Read the model definition and answer for the solid it produces. Units are mm, in the model's axes. A direction names the side the tool comes from. Round coordinates to 2 decimals unless told otherwise and drop trailing zeros. Write each loop counter-clockwise with the first axis right and the second up, starting at its lowest first coordinate (ties: lowest second). Pieces come first, ordered by that corner, then holes. Notation, with made-up numbers: (75, 50) -> (107, 50) arc R27 ccw to (107, 87) -> close; hole circle Ø11 at (64, 7.5). An arc over 180 degrees is marked (long way). Return JSON: item names as keys, results as strings. Group by question number.
(1) For faces 4 (the flat face through (49, 27, -44)), 5 (the flat face through (39, 16, -14.9)), 6 (the flat face through (93, 14, -42)), 7 (the flat face through (8, 6.4, -32)), 8 (the flat face through (72, 6.4, -7)), determine the directions among +Z, -Z, +X, -X, +Y, -Y from which every point of the face is accessible in a straight line to the end or side of a thin tool.
(2) The mould has two halves that part along Y. Classify faces 1 (the flat face through (0, 5, -33)), 2 (the flat face through (8, 14, -21.5)), 3 (the flat face through (50, 25, -7)): released by +Y, released by -Y, zero draft, split by the parting line, or undercut.
(3) A cutting plane is placed at A-A on z = -77. Give the vertices of the cut face in (x, y), then the cut area to 3 significant figures.
(4) A cutting plane is placed at D-D on y = 14. State how many separate pieces and enclosed holes the cut face has, then the cut area to 3 significant figures.
(5) Straight lines are drawn through the part: line 1 (X direction, y = 22, z = -9); line 2 (Z direction, x = 75, y = 5.5); line 3 (Y direction, x = 95.5, z = -25). For each, find the intervals that lie inside material, in ascending order.
(6) A cutting plane is placed at C-C on y = 32. Give the vertices of the cut face in (x, z), then the cut area to 4 significant figures.
(7) Given pin 1 (16.5 mm diameter, centred on x = 29, z = -6, fed in from -Y); pin 2 (5 mm diameter, centred on x = 77, z = -45, fed in from +Y); pin 3 (1.5 mm diameter, centred on x = 49.5, z = -70.5, fed in from -Y); pin 4 (2.5 mm diameter, centred on x = 48, z = -20, fed in from +Y), each flat-ended and moving along its own axis, determine where each tip first touches the part or whether it passes through.
(8) A cutting plane is placed at B-B on x = 30. Give the vertices of the cut face in (y, z).
```python
from build123d import *

# Parameters (mm, degrees)
CROQUIS1_W              = 100
CROQUIS1_H              = 49
SALIENTE_EXTRUIR1_DEPTH = 40
CROQUIS2_W              = 70
CROQUIS2_H              = 29
CORTAR_EXTRUIR1_DEPTH   = 35
CORTAR_EXTRUIR2_DEPTH   = 14.9
CORTAR_EXTRUIR4_DEPTH   = 119.325821358
CROQUIS6_W              = 20.5
CROQUIS6_H              = 16.2
CORTAR_EXTRUIR6_DEPTH   = 119.325821358
CROQUIS7_W              = 58
CROQUIS7_H              = 18
SALIENTE_EXTRUIR2_DEPTH = 16
CROQUIS8_W              = 54
CROQUIS8_H              = 14
CORTAR_EXTRUIR7_DEPTH   = 16
ENVOLVER2_START         = -2.5
ENVOLVER2_DEPTH         = 2.5
CROQUIS11_W             = 75
CROQUIS11_H             = 10
SALIENTE_EXTRUIR3_DEPTH = 51
CROQUIS12_W             = 67
CROQUIS12_H             = 52
CORTAR_EXTRUIR8_DEPTH   = 5
CROQUIS13_W             = 71
CROQUIS13_H             = 1.5
CORTAR_EXTRUIR9_DEPTH   = 54
CROQUIS14_W             = 20
CROQUIS14_H             = 12
CORTAR_EXTRUIR10_DEPTH  = 5
CORTAR_EXTRUIR11_REACH  = 148.969
CROQUIS5_W              = 20.5
CROQUIS5_H              = 16.2


# Read off the part's stored shape, not the designer's step: Envolver2
with BuildPart() as part:
    # Croquis1 → Saliente-Extruir1 (new body)
    with BuildSketch(Plane(origin=(0, 0, 0), x_dir=(1, 0, 0), z_dir=(0, 1, 0))):
        with Locations((50, 24.5)):
            Rectangle(CROQUIS1_W, CROQUIS1_H)
    extrude(amount=SALIENTE_EXTRUIR1_DEPTH)

    # Croquis2 → Cortar-Extruir1 (cut)
    with BuildSketch(Plane(origin=(0, 40, 0), x_dir=(1, 0, 0), z_dir=(0, 1, 0))):
        with Locations((50, 29.5)):
            Rectangle(CROQUIS2_W, CROQUIS2_H)
    extrude(amount=-CORTAR_EXTRUIR1_DEPTH, mode=Mode.SUBTRACT)

    # Croquis3 → Cortar-Extruir2 (cut)
    with BuildSketch(Plane.XY):
        Polygon((15, 5), (15, 25), (85, 25), (85, 5), (100, 5), (100, 40), (0, 40), (0, 5), align=None)
    extrude(amount=-CORTAR_EXTRUIR2_DEPTH, mode=Mode.SUBTRACT)

    # Croquis4 → Cortar-Extruir4 (cut, through all)
    with BuildSketch(Plane.ZY):
        Polygon((-44, 25), (-19, 25), (-19, 5), (-14.9, 5), (-14.9, 40), (-44, 40), align=None)
    extrude(amount=-CORTAR_EXTRUIR4_DEPTH, mode=Mode.SUBTRACT)

    # Croquis6 → Cortar-Extruir6 (cut, through all)
    with BuildSketch(Plane(origin=(100, 0, 0), x_dir=(0, 0, -1), z_dir=(1, 0, 0))):
        with Locations((31.75, 14.5)):
            Rectangle(CROQUIS6_W, CROQUIS6_H)
    extrude(amount=-CORTAR_EXTRUIR6_DEPTH, mode=Mode.SUBTRACT)

    # Croquis7 → Saliente-Extruir2 (add)
    with BuildSketch(Plane(origin=(0, 5, 0), x_dir=(1, 0, 0), z_dir=(0, 1, 0))):
        with Locations((50, 35)):
            Rectangle(CROQUIS7_W, CROQUIS7_H)
    extrude(amount=SALIENTE_EXTRUIR2_DEPTH)

    # Croquis8 → Cortar-Extruir7 (cut)
    with BuildSketch(Plane(origin=(0, 21, 0), x_dir=(1, 0, 0), z_dir=(0, 1, 0))):
        with Locations((50, 35)):
            Rectangle(CROQUIS8_W, CROQUIS8_H)
    extrude(amount=-CORTAR_EXTRUIR7_DEPTH, mode=Mode.SUBTRACT)

    # Envolver2 outline → Envolver2 (cut)
    # profile 1 of 3: a face of its own
    with BuildSketch(Plane(origin=(0, 5, 0), x_dir=(1, 0, 0), z_dir=(0, 1, 0)).offset(ENVOLVER2_START)):
        with BuildLine():
            add(Edge.make_bspline(
                [(44.845927513, 22.682039813), (44.880502524, 22.681581101), (44.94779002, 22.680688388), (45.045978034, 22.678103561), (45.138406194, 22.671034857), (45.225422346, 22.663758255), (45.306894242, 22.652117669), (45.382891805, 22.638865253), (45.453428219, 22.622573117), (45.519399834, 22.604194379), (45.582065701, 22.58175166), (45.642294727, 22.553081251), (45.700763218, 22.518735345), (45.757273689, 22.477750733), (45.813128977, 22.432374893), (45.865885411, 22.37921084), (45.918377238, 22.321807714), (45.967578278, 22.25830401), (46.01447324, 22.191680732), (46.054376208, 22.120908747), (46.088223994, 22.047966819), (46.117214563, 21.973058038), (46.136979973, 21.894799291), (46.154181469, 21.814812457), (46.162464556, 21.732060085), (46.163897144, 21.676148523), (46.164618555, 21.647993057)],
                knots=[0, 0, 0, 0, 0.054369818, 0.105810783, 0.1543913, 0.200099433, 0.243069893, 0.283740822, 0.321360744, 0.356845277, 0.391373506, 0.42587086, 0.461574928, 0.497826917, 0.535543491, 0.574581255, 0.615459073, 0.657779879, 0.700797841, 0.743450957, 0.785305491, 0.827181235, 0.869502041, 0.912065543, 0.955718718, 1, 1, 1, 1], degree=3))
            Line((44.845927513, 22.682039813), (43.424314244, 22.682039813))
            Line((43.424314244, 22.682039813), (42.805172718, 18.976839617))
            Line((42.805172718, 18.976839617), (43.469342719, 18.976839617))
            Line((43.469342719, 18.976839617), (43.718607489, 20.469211918))
            Line((43.718607489, 20.469211918), (44.603095383, 20.469211918))
            Line((44.603095383, 20.469211918), (45.04292709, 18.976839617))
            Line((45.04292709, 18.976839617), (45.752929645, 18.976839617))
            Line((45.752929645, 18.976839617), (45.28977962, 20.548011749))
            add(Edge.make_bspline(
                [(46.164618555, 21.647993057), (46.164091676, 21.617670303), (46.163039403, 21.5571103), (46.151744736, 21.467468845), (46.13622668, 21.379126232), (46.112503265, 21.292592771), (46.082048693, 21.207680933), (46.044780457, 21.124441143), (46.001130757, 21.043108672), (45.951712013, 20.9635574), (45.895224481, 20.887990565), (45.830214645, 20.819272615), (45.758276279, 20.757071565), (45.678885267, 20.701205138), (45.592072867, 20.652370985), (45.497799172, 20.610367641), (45.396617343, 20.574987864), (45.325850603, 20.557119534), (45.28977962, 20.548011749)],
                knots=[0, 0, 0, 0, 0.059520551, 0.118873267, 0.177208837, 0.235565778, 0.294841411, 0.354222133, 0.414510544, 0.476000381, 0.538010758, 0.599455515, 0.661405537, 0.724496825, 0.78978963, 0.856706752, 0.926961053, 1, 1, 1, 1], degree=3))
        make_face()
        with BuildLine():
            add(Edge.make_bspline(
                [(44.743809366, 21.03528417), (44.778129381, 21.03600119), (44.843652036, 21.0373701), (44.937526666, 21.044910102), (45.022020151, 21.059216882), (45.097465695, 21.079213334), (45.164300411, 21.104537257), (45.221481868, 21.136836672), (45.270624581, 21.17399479), (45.32077283, 21.232312946), (45.36864261, 21.310567266), (45.413007527, 21.407196099), (45.438530205, 21.507321555), (45.442292151, 21.574957755), (45.444162962, 21.608593141)],
                knots=[0, 0, 0, 0, 0.099664188, 0.190275618, 0.273183536, 0.348129931, 0.416633313, 0.480054439, 0.538277477, 0.594505454, 0.702244126, 0.80362549, 0.902343236, 1, 1, 1, 1], degree=3))
            Line((44.743809366, 21.03528417), (43.812684837, 21.03528417))
            Line((43.812684837, 21.03528417), (43.993602816, 22.115967561))
            Line((43.993602816, 22.115967561), (44.735768567, 22.115967561))
            add(Edge.make_bspline(
                [(45.444162962, 21.608593141), (45.443321191, 21.636863214), (45.441681994, 21.691914124), (45.421908744, 21.770970842), (45.392768442, 21.844328967), (45.35019923, 21.909220717), (45.300609579, 21.965653441), (45.246923641, 22.013950522), (45.187891151, 22.050903022), (45.122329195, 22.077622199), (45.046506806, 22.09459194), (44.957252302, 22.107151834), (44.85196106, 22.115045121), (44.776255138, 22.115646142), (44.735768567, 22.115967561)],
                knots=[0, 0, 0, 0, 0.084973229, 0.165470167, 0.24404472, 0.32176826, 0.397881214, 0.469968558, 0.538528016, 0.606605512, 0.682202732, 0.771959831, 0.878046995, 1, 1, 1, 1], degree=3))
        make_face(mode=Mode.SUBTRACT)
    # profile 2 of 3: a face of its own
    with BuildSketch(Plane(origin=(0, 5, 0), x_dir=(1, 0, 0), z_dir=(0, 1, 0)).offset(ENVOLVER2_START)):
        Polygon((46.976739258, 22.682039813), (46.357597732, 18.976839617), (48.79395984, 18.976839617), (48.892057588, 19.542911869), (47.113432841, 19.542911869), (47.285505941, 20.572134146), (48.696666171, 20.572134146), (48.78913536, 21.138206398), (47.379583289, 21.138206398), (47.54281151, 22.115967561), (49.257109864, 22.115967561), (49.355207612, 22.682039813), align=None)
    # profile 3 of 3: a face of its own
    with BuildSketch(Plane(origin=(0, 5, 0), x_dir=(1, 0, 0), z_dir=(0, 1, 0)).offset(ENVOLVER2_START)):
        Polygon((50.984273497, 22.682039813), (49.96148386, 22.682039813), (49.342342334, 18.976839617), (49.858561632, 18.976839617), (50.417397165, 22.321007936), (50.952914381, 18.976839617), (51.313946257, 18.976839617), (52.891551028, 22.350758892), (52.327086936, 18.976839617), (52.991256936, 18.976839617), (53.611202541, 22.682039813), (52.559466028, 22.682039813), (51.387921608, 20.172506434), align=None)
    extrude(amount=ENVOLVER2_DEPTH, mode=Mode.SUBTRACT)

    # Croquis11 → Saliente-Extruir3 (add)
    with BuildSketch(Plane(origin=(0, 0, -49), x_dir=(-1, 0, 0), z_dir=(0, 0, -1))):
        with Locations((-50, 35)):
            Rectangle(CROQUIS11_W, CROQUIS11_H)
    extrude(amount=SALIENTE_EXTRUIR3_DEPTH)

    # Croquis12 → Cortar-Extruir8 (cut)
    with BuildSketch(Plane(origin=(0, 40, 0), x_dir=(1, 0, 0), z_dir=(0, 1, 0))):
        with Locations((50, 70)):
            Rectangle(CROQUIS12_W, CROQUIS12_H)
    extrude(amount=-CORTAR_EXTRUIR8_DEPTH, mode=Mode.SUBTRACT)

    # Croquis13 → Cortar-Extruir9 (cut)
    with BuildSketch(Plane.XY.offset(-44)):
        with Locations((50, 37.5)):
            Rectangle(CROQUIS13_W, CROQUIS13_H)
    extrude(amount=-CORTAR_EXTRUIR9_DEPTH, mode=Mode.SUBTRACT)

    # Croquis14 → Cortar-Extruir10 (cut)
    with BuildSketch(Plane(origin=(0, 35, 0), x_dir=(1, 0, 0), z_dir=(0, 1, 0))):
        with Locations((50.5, 81)):
            Rectangle(CROQUIS14_W, CROQUIS14_H)
    extrude(amount=-CORTAR_EXTRUIR10_DEPTH, mode=Mode.SUBTRACT)

    # Croquis5 → Cortar-Extruir11 (cut, up to next)
    with BuildSketch(Plane.XY, mode=Mode.PRIVATE) as cortar_extruir11_sk1:
        with Locations((27.5, 14.5)):
            Rectangle(CROQUIS5_W, CROQUIS5_H)
    cortar_extruir11_tool1 = extrude(cortar_extruir11_sk1.sketch, amount=-CORTAR_EXTRUIR11_REACH, mode=Mode.PRIVATE) & part.part
    # Croquis5 → Cortar-Extruir11 (cut, up to next)
    with BuildSketch(Plane.XY, mode=Mode.PRIVATE) as cortar_extruir11_sk2:
        with Locations((50, 14.5)):
            Rectangle(CROQUIS5_W, CROQUIS5_H)
    cortar_extruir11_tool2 = extrude(cortar_extruir11_sk2.sketch, amount=-CORTAR_EXTRUIR11_REACH, mode=Mode.PRIVATE) & part.part
    # Croquis5 → Cortar-Extruir11 (cut, up to next)
    with BuildSketch(Plane.XY, mode=Mode.PRIVATE) as cortar_extruir11_sk3:
        with Locations((72.5, 14.5)):
            Rectangle(CROQUIS5_W, CROQUIS5_H)
    cortar_extruir11_tool3 = extrude(cortar_extruir11_sk3.sketch, amount=-CORTAR_EXTRUIR11_REACH, mode=Mode.PRIVATE) & part.part
    add(cortar_extruir11_tool1.solids().sort_by_distance((27.5, 14.5, 0))[0], mode=Mode.SUBTRACT)
    add(cortar_extruir11_tool2.solids().sort_by_distance((50, 14.5, 0))[0], mode=Mode.SUBTRACT)
    add(cortar_extruir11_tool3.solids().sort_by_distance((72.5, 14.5, 0))[0], mode=Mode.SUBTRACT)


solid = part.part
```
Checks:
{
 "1": {"face 4": "+Y", "face 5": "+X, -X, +Y", "face 6": "+X", "face 7": "-X", "face 8": "+Z"},
 "2": {"face 1": "zero draft", "face 2": "undercut", "face 3": "released by +Y"},
 "3": {"outline": "(12.5, 30) -> (40.5, 30) -> (40.5, 35) -> (16.5, 35) -> (16.5, 36.75) -> (14.5, 36.75) -> (14.5, 38.25) -> (16.5, 38.25) -> (16.5, 40) -> (12.5, 40) -> close; (60.5, 30) -> (87.5, 30) -> (87.5, 40) -> (83.5, 40) -> (83.5, 38.25) -> (85.5, 38.25) -> (85.5, 36.75) -> (83.5, 36.75) -> (83.5, 35) -> (60.5, 35) -> close", "area": "309 mm^2"},
 "4": {"separate pieces": "7", "enclosed holes": "1", "area": "1,050 mm^2"},
 "5": {"line 1": "x = 15 to 17.25, 37.75 to 39.75, 60.25 to 62.25, 82.75 to 85", "line 2": "z = -49 to -42, -28 to -26, -14.9 to 0", "line 3": "y = 0 to 6.4, 22.6 to 25"},
 "6": {"outline": "(0, -49) -> (12.5, -49) -> (12.5, -100) -> (87.5, -100) -> (87.5, -49) -> (100, -49) -> (100, -44) -> (0, -44) -> close; hole (40.5, -87) -> (60.5, -87) -> (60.5, -75) -> (40.5, -75) -> close", "area": "4,085 mm^2"},
 "7": {"pin 1": "stops at y = 0", "pin 2": "stops at y = 35", "pin 3": "stops at y = 30", "pin 4": "stops at y = 5"},
 "8": {"outline": "(0, -49) -> (30, -49) -> (30, -100) -> (40, -100) -> (40, -96) -> (38.25, -96) -> (38.25, -98) -> (36.75, -98) -> (36.75, -96) -> (35, -96) -> (35, -44) -> (21, -44) -> (21, -42) -> (5, -42) -> (5, -28) -> (21, -28) -> (21, -26) -> (5, -26) -> (5, -14.9) -> (6.4, -14.9) -> (6.4, 0) -> (0, 0) -> close; (22.6, -14.9) -> (25, -14.9) -> (25, 0) -> (22.6, 0) -> close"}
}
